```python
from build123d import *

# Parameters (mm, degrees)
SKETCH1_W           = 32
SKETCH1_H           = 24
BOSS_EXTRUDE1_DEPTH = 16.3
SKETCH2_W           = 50
SKETCH2_H           = 28.3
BOSS_EXTRUDE2_DEPTH = 3.2
FILLET1_R           = 3.5
CHAMFER1_SIZE       = 5
CHAMFER2_SIZE       = 9
SKETCH3_R           = 1.6
CUT_EXTRUDE1_DEPTH  = 3.2


with BuildPart() as part:
    # Sketch1 → Boss-Extrude1 (new body)
    with BuildSketch(Plane(origin=(0, 0, 0), x_dir=(1, 0, 0), z_dir=(0, 1, 0))):
        Rectangle(SKETCH1_W, SKETCH1_H)
    extrude(amount=BOSS_EXTRUDE1_DEPTH)

    # Sketch2 → Boss-Extrude2 (add)
    with BuildSketch(Plane(origin=(0, 16.3, 0), x_dir=(1, 0, 0), z_dir=(0, 1, 0))):
        Rectangle(SKETCH2_W, SKETCH2_H)
    extrude(amount=BOSS_EXTRUDE2_DEPTH)

    # Fillet1
    fillet1_edges = [part.edges().sort_by_distance(p)[0] for p in [
        (16, 8.15, 12),
        (-16, 8.15, 12),
    ]]
    fillet(fillet1_edges, radius=FILLET1_R)

    # Chamfer1
    chamfer1_edges = [part.edges().sort_by_distance(p)[0] for p in [
        (-16, 8.15, -12),
        (16, 8.15, -12),
    ]]
    chamfer(chamfer1_edges, length=CHAMFER1_SIZE)

    # Chamfer2
    chamfer2_edges = [part.edges().sort_by_distance(p)[0] for p in [
        (25, 17.9, 14.15),
        (25, 17.9, -14.15),
        (-25, 17.9, -14.15),
        (-25, 17.9, 14.15),
    ]]
    chamfer(chamfer2_edges, length=CHAMFER2_SIZE)

    # Sketch3 → Cut-Extrude1 (cut)
    with BuildSketch(Plane(origin=(0, 19.5, 0), x_dir=(1, 0, 0), z_dir=(0, 1, 0))):
        with Locations(Location((-20, 0, 0), (0, 0, 270))):
            Circle(SKETCH3_R)
        with Locations(Location((20, 0, 0), (0, 0, 90))):
            Circle(SKETCH3_R)
    extrude(amount=-CUT_EXTRUDE1_DEPTH, mode=Mode.SUBTRACT)


solid = part.part
```
Here's how the part is built. I have some questions about the finished solid (model axes, mm). A direction names the side the tool comes from. Coordinates: 2 decimals unless noted, no trailing zeros. Order: outer loops, then holes, each group sorted by start corner. A loop starts at its lowest first (then second) coordinate and runs counter-clockwise, first axis right, second up.
1) Imagine slicing it at C-C on y = 4.5. List the corners of the cut face in (x, z) for me.
2) Imagine slicing it at A-A on x = -20. List the corners of the cut face in (y, z) for me, and give its area (3 significant figures).
3) We'd pull the mould along Z, two halves only. Please class faces 1 (the face through (18.414, 17.922, 0.208)), 2 (the face through (-0.3, 16.3, 12.4)), 3 (the face through (-18.414, 17.922, -0.208)), 4 (the face through (-14.95, 8.26, 11)): +Z half, -Z half, draft (parallel to the pull), parting line (faces both ways), or undercut.
4) Which directions (+Z, -Z, +X, -X, +Y, -Y) give clear straight access to the entire face, cutting with the end or side of a thin tool? Please do faces 5 (the face through (-13, 8, -10)), 6 (the face through (0, 8, -12)), 7 (the face through (14.95, 8.26, 11)), 8 (the face through (13, 8, -10)), 9 (the face through (16, 8, 1)).
5) Will these pins go through, and if not, where does the flat tip stop? pin 1 (8 mm diameter, centred on x = -0.5, y = 4, fed in from +Z); pin 2 (5 mm diameter, centred on x = -20, z = -3.5, fed in from -Y); pin 3 (5 mm diameter, centred on x = -5, y = 9, fed in from -Z); pin 4 (6 mm diameter, centred on x = -19.5, y = 8.5, fed in from +Z).
6) I need wall thicknesses on line 1 (X direction, y = 17.05, z = 0); line 2 (X direction, y = 18.25, z = -0.75); line 3 (X direction, y = 15.5, z = 1). Which ranges of each line are inside material? Lowest first, please.
7) Imagine slicing it at D-D on z = -9.25. List the corners of the cut face in (x, y) for me, and give its area (3 significant figures).
8) Imagine slicing it at B-B on z = 0. List the corners of the cut face in (x, y) for me, and give its area (3 significant figures).
Response values:
1. outline: (-16, -7) - (-11, -12) - (11, -12) - (16, -7) - (16, 8.5) arc R3.5 ccw to (12.5, 12) - (-12.5, 12) arc R3.5 ccw to (-16, 8.5) - close
2. outline: (16.3, -10.15) - (19.5, -10.15) - (19.5, -1.6) - (16.3, -1.6) - close; (16.3, 1.6) - (19.5, 1.6) - (19.5, 10.15) - (16.3, 10.15) - close
2. area: 54.7 mm2
3. face 1: undercut
3. face 2: draft
3. face 3: undercut
3. face 4: +Z half
4. face 5: -Z, -X, -Y
4. face 6: -Z, +X, -X, -Y
4. face 7: +Z, +X, -Y
4. face 8: -Z, +X, -Y
4. face 9: +Z, -Z, +X, -Y
5. pin 1: stops at z = 12
5. pin 2: stops at y = 16.3
5. pin 3: stops at z = -12
5. pin 4: passes through
6. line 1: x = -25 to -21.6, -18.4 to 18.4, 21.6 to 25
6. line 2: x = -25 to -21.41, -18.59 to 18.59, 21.41 to 25
6. line 3: x = -16 to 16
7. outline: (-20.9, 16.3) - (-13.75, 16.3) - (-13.75, 0) - (13.75, 0) - (13.75, 16.3) - (20.9, 16.3) - (20.9, 19.5) - (-20.9, 19.5) - close
7. area: 582 mm2
8. outline: (-25, 16.3) - (-21.6, 16.3) - (-21.6, 19.5) - (-25, 19.5) - close; (-18.4, 16.3) - (-16, 16.3) - (-16, 0) - (16, 0) - (16, 16.3) - (18.4, 16.3) - (18.4, 19.5) - (-18.4, 19.5) - close; (21.6, 16.3) - (25, 16.3) - (25, 19.5) - (21.6, 19.5) - close
8. area: 661 mm2
